from build123d import *

# Parameters (mm, degrees)
F0_R     = 18
F1_DEPTH = 9.5
F2_R     = 15
F3_DEPTH = 5
F4_R     = 6
F5_DEPTH = 5
F6_SIZE  = 1
F8_R     = 1
F9_R     = 1


# Not quite as in the source:
# - a fillet or chamfer that OpenCascade refuses, or shapes differently, is made with other operations: its cross-section is extruded or revolved along the edge and cut away or added


with BuildPart() as f1:
    # F0 (on Top) → F1 (new body)
    with BuildSketch(Plane.XY):
        Circle(F0_R)
    extrude(amount=F1_DEPTH)

    # F2 (on face) → F3 (cut)
    with BuildSketch(Plane.XY.offset(9.5)):
        Circle(F2_R)
    extrude(amount=-F3_DEPTH, mode=Mode.SUBTRACT)

    # F4 (on Top) → F5 (cut)
    with BuildSketch(Plane.XY):
        Circle(F4_R)
    extrude(amount=F5_DEPTH, mode=Mode.SUBTRACT)

    # F6
    f6_edges = [f1.edges().sort_by_distance(p)[0] for p in [
        (-6, 0, 4.5),
    ]]
    chamfer(f6_edges, length=F6_SIZE)

    # F7: chamfer of 5 on 1 edges, made by hand

    # F7_s1 → F7_t2 (revolve, cut)
    with BuildSketch(Plane.XZ):
        Polygon((18, 4.5), (13, 9.5), (18, 9.5), align=None)
    revolve(axis=Axis((0, 0, 9.5), (0, 0, 1)), mode=Mode.SUBTRACT)

    # F8
    f8_edges = [f1.edges().sort_by_distance(p)[0] for p in [
        (-18, 0, 4.5),
    ]]
    fillet(f8_edges, radius=F8_R)

    # F9
    f9_edges = [f1.edges().sort_by_distance(p)[0] for p in [
        (-18, 0, 0),
    ]]
    fillet(f9_edges, radius=F9_R)


solid = f1.part
Work out the finished part from the listing and answer in its coordinate system (mm). Round coordinates to 2 decimals unless told otherwise and drop trailing zeros. Write each loop counter-clockwise with the first axis right and the second up, starting at its lowest first coordinate (ties: lowest second). Pieces come first, ordered by that corner, then holes. Notation, with made-up numbers: M 33,-29 L 68,-29 A7 ccw 68,-21 Z; hole C 3,15 d7. An arc over 180 degrees is marked long. Use a Markdown table: item, result.
1) Determine the mould class of faces 1 (the face through (7, 0, 0)), 2 (the face through (-6, 0, 2)), 3 (the face through (-14.284, -10.953, 2.521)) for opening direction X: pulls with the +X half, pulls with the -X half, needs draft (parallel to the pull), parting line crosses it, or undercut.
Taken from the geometry:
| item | result |
|---|---|
| face 1 | needs draft |
| face 2 | undercut |
| face 3 | parting line crosses it |
2) The part is cut by section A-A on z = 1.5. Give the vertices of the cut face in (x, y).
Taken from the geometry:
| item | result |
|---|---|
| outline | C 0,0 d36; hole C 0,0 d12 |
3) Flat-ended cylindrical pins translate along their axes: pin 1 (4 mm diameter, centred on y = 8.5, z = 6.5, fed in from -X); pin 2 (2 mm diameter, centred on x = -1.5, y = -11, fed in from +Z). Find the tip coordinate at first contact, or state that the pin passes through.
Taken from the geometry:
| item | result |
|---|---|
| pin 1 | stops at x = -16.07 |
| pin 2 | stops at z = 4.5 |
4) Consider line 1 (Y direction, x = 0, z = 1.6); line 2 (Y direction, x = 0, z = 5.4); line 3 (Z direction, x = -8.5, y = 10). Determine where each line is inside the solid, lowest interval first. Write a range as [from, to].
Taken from the geometry:
| item | result |
|---|---|
| line 1 | y = [-18, -6], [6, 18] |
| line 2 | y = [-17.1, -15], [15, 17.1] |
| line 3 | z = [0, 4.5] |
